Can you work these out from the drawing? Everything is in mm from the part's minimum corner. Round coordinates to 2 decimals unless told otherwise and drop trailing zeros. Loops run counter-clockwise (first coordinate to the right, second up) from the corner with the lowest first, then second, coordinate; pieces in that order, holes last. Notation, with made-up numbers: M -30.75,82.25 L -7.75,82.25 A16 ccw -7.75,93.25 Z; hole C 11.5,18.5 d10. An arc over 180 degrees is marked long. Return JSON: item names as keys, results as strings. Group by question number.
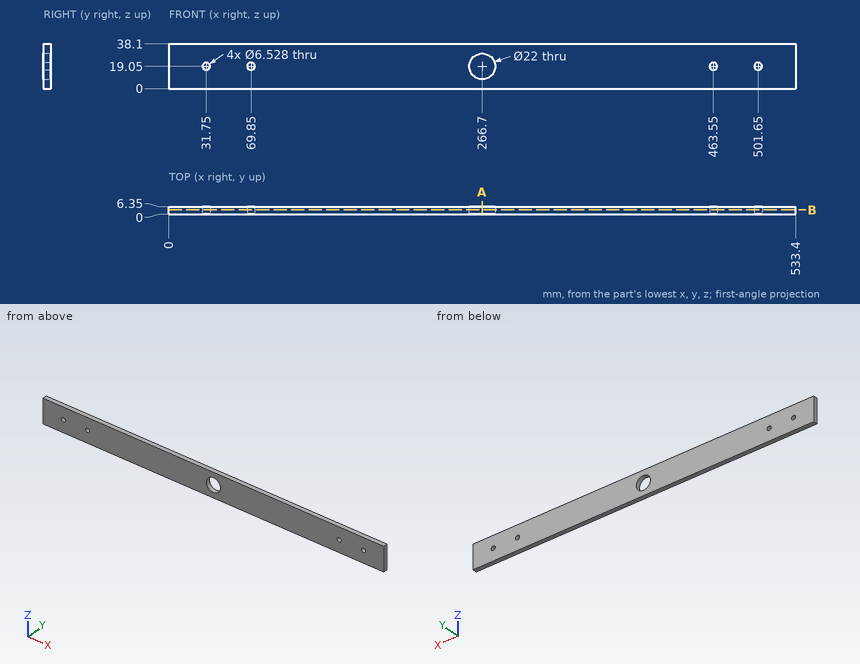
1. If we section it at A-A, the plane x = 266.7: Please give me the cut outline in (y, z), then the cut area to 3 significant figures.
2. If we section it at B-B, the plane y = 3.75: Please give me the cut outline in (x, z), then the cut area to 3 significant figures.
3. I need wall thicknesses on probe 1 along X at (y, z) = (0.75, 19); probe 2 along Z at (x, y) = (463.55, 3.5); probe 3 along Z at (x, y) = (266.7, 2.75). Which ranges of each line are inside material? Lowest first, please.
Geometry results:
{
 "1": {"outline": "M 0,0 L 6.35,0 L 6.35,8.05 L 0,8.05 Z; M 0,30.05 L 6.35,30.05 L 6.35,38.1 L 0,38.1 Z", "area": "102 mm^2"},
 "2": {"outline": "M 0,0 L 533.4,0 L 533.4,38.1 L 0,38.1 Z; hole C 31.75,19.05 d6.53; hole C 69.85,19.05 d6.53; hole C 266.7,19.05 d22; hole C 463.55,19.05 d6.53; hole C 501.65,19.05 d6.53", "area": "19,800 mm^2"},
 "3": {"probe 1": "0 to 28.49, 35.01 to 66.59, 73.11 to 255.7, 277.7 to 460.29, 466.81 to 498.39, 504.91 to 533.4", "probe 2": "0 to 15.79, 22.31 to 38.1", "probe 3": "0 to 8.05, 30.05 to 38.1"}
}
